Here's how the part is built. I have some questions about the finished solid (model axes, mm). A direction names the side the tool comes from. Give positions to 0.01 mm unless a question says otherwise; leave off trailing zeros. Loops run counter-clockwise (first coordinate to the right, second up) from the corner with the lowest first, then second, coordinate; pieces in that order, holes last. Notation, with made-up numbers: M 77.25,-4.75 L 86.25,-4.75 A17 cw 86.25,20.25 Z; hole C 34.25,-2.75 d2. An arc over 180 degrees is marked long. Answer as CSV lines item,"result". Start each with the question number.
Item 1: If I drill on line 1 along Y through (x, z) = (1, -1.75); line 2 along Y through (x, z) = (-0.75, 2); line 3 along Y through (x, z) = (4, -5), over which ranges is the centre line in solid material (lowest first)? Write a range as from..to.
Item 2: I want a section at D-D on y = 5.25. List the corners of the cut face in (x, z) for me.
Item 3: For faces 1 (the flat face through (-1.9, 7, 0)), 2 (the flat face through (-5.5, 1.6, -5.5)), which set-ups out of +Z, -Z, +X, -X, +Y, -Y let a thin tool reach every point of the face, with its end or its side?
Item 4: I want a section at A-A on z = 0. List the corners of the cut face in (x, y) for me.
Item 5: Will these pins go through, and if not, where does the flat tip stop? P1, Ø3, axis at x = -1, z = 0.5, coming from the -Y side; P2, Ø1.2, axis at x = -6.5, y = 0, coming from the -Z side; P3, Ø0.7, axis at x = 0, y = 5.5, coming from the +Z side.
Item 6: I want a section at B-B on x = 0. List the corners of the cut face in (y, z) for me, plus the area to 3 significant figures.
Item 7: I want a section at C-C on y = 0.5. List the corners of the cut face in (x, z) for me, plus the area to 3 significant figures.
Item 8: If we mould it in two halves opening along Y, with no side actions, what happens to faces 3 (the flat face through (3, 3.3, -3)), 4 (the flat face through (-1.6, 5, 0)), 5 (the flat face through (0, 0, 0)), 6 (the cylindrical face through (-2.038, 3.99, -2.658))? For each: released by +Y, released by -Y, zero draft, split by the parting line, or undercut.
from build123d import *

# Parameters (mm, degrees)
BOSS_EXTRUDE1_DEPTH = 3.3
BOSS_EXTRUDE2_START = 3.3
SKETCH3_R           = 3.35
BOSS_EXTRUDE2_DEPTH = 1.4
BOSS_EXTRUDE3_START = 4.7
SKETCH3_3_W         = 3.2
SKETCH3_3_H         = 3.2
BOSS_EXTRUDE3_DEPTH = 1.4
BOSS_EXTRUDE4_START = 6.1
SKETCH3_4_W         = 3.8
SKETCH3_4_H         = 3.8
BOSS_EXTRUDE4_DEPTH = 1.2
BOSS_EXTRUDE5_START = 2.5
BOSS_EXTRUDE5_DEPTH = 1
BOSS_EXTRUDE6_START = -2.5
BOSS_EXTRUDE6_DEPTH = 1


with BuildPart() as part:
    # Sketch1 → Boss-Extrude1 (new body)
    with BuildSketch(Plane(origin=(0, 0, 0), x_dir=(1, 0, 0), z_dir=(0, 1, 0))):
        Polygon((-5, 6), (-6, 5), (-6, -5), (-5, -6), (5, -6), (6, -5), (6, 5), (5, 6), align=None)
    extrude(amount=BOSS_EXTRUDE1_DEPTH)

    # Sketch3 → Boss-Extrude2 (add)
    with BuildSketch(Plane(origin=(0, 0, 0), x_dir=(1, 0, 0), z_dir=(0, 1, 0)).offset(BOSS_EXTRUDE2_START)):
        with Locations(Location((0, 0, 0), (0, 0, 270))):
            Circle(SKETCH3_R)
    extrude(amount=BOSS_EXTRUDE2_DEPTH)

    # Sketch3<3> → Boss-Extrude3 (add)
    with BuildSketch(Plane(origin=(0, 0, 0), x_dir=(1, 0, 0), z_dir=(0, 1, 0)).offset(BOSS_EXTRUDE3_START)):
        Rectangle(SKETCH3_3_W, SKETCH3_3_H)
    extrude(amount=BOSS_EXTRUDE3_DEPTH)

    # Sketch3<4> → Boss-Extrude4 (add)
    with BuildSketch(Plane(origin=(0, 0, 0), x_dir=(1, 0, 0), z_dir=(0, 1, 0)).offset(BOSS_EXTRUDE4_START)):
        Rectangle(SKETCH3_4_W, SKETCH3_4_H)
    extrude(amount=BOSS_EXTRUDE4_DEPTH)

    # Sketch4 → Boss-Extrude5 (add)
    with BuildSketch(Plane.XY.offset(BOSS_EXTRUDE5_START)):
        Polygon((6, 1.543469882), (7.05, -1.890925367), (6.35, -3.028306733), (6.35, -3.5), (6.25, -3.5), (6.25, -3), (6.941165312, -1.876973505), (6, 1.20143952), align=None)
        Polygon((-6.941165312, -1.876973505), (-6, 1.20143952), (-6, 1.543469882), (-7.05, -1.890925367), (-6.35, -3.028306733), (-6.35, -3.5), (-6.25, -3.5), (-6.25, -3), align=None)
    extrude(amount=BOSS_EXTRUDE5_DEPTH)

    # Sketch4<2> → Boss-Extrude6 (add)
    with BuildSketch(Plane.XY.offset(BOSS_EXTRUDE6_START)):
        Polygon((6, 1.543469882), (7.05, -1.890925367), (6.35, -3.028306733), (6.35, -3.5), (6.25, -3.5), (6.25, -3), (6.941165312, -1.876973505), (6, 1.20143952), align=None)
        Polygon((-6.941165312, -1.876973505), (-6, 1.20143952), (-6, 1.543469882), (-7.05, -1.890925367), (-6.35, -3.028306733), (-6.35, -3.5), (-6.25, -3.5), (-6.25, -3), align=None)
    extrude(amount=-BOSS_EXTRUDE6_DEPTH)


solid = part.part
Result:
1,line 1,"0..4.7, 6.1..7.3"
1,line 2,"0..4.7"
1,line 3,"0..3.3"
2,outline,"M -1.6,-1.6 L 1.6,-1.6 L 1.6,1.6 L -1.6,1.6 Z"
3,face 1,"+Z, -Z, -X, +Y"
3,face 2,"-Z, -X, +Y, -Y"
4,outline,"M -6,0 L 6,0 L 6,3.3 L 3.35,3.3 L 3.35,4.7 L 1.6,4.7 L 1.6,6.1 L 1.9,6.1 L 1.9,7.3 L -1.9,7.3 L -1.9,6.1 L -1.6,6.1 L -1.6,4.7 L -3.35,4.7 L -3.35,3.3 L -6,3.3 Z"
5,P1,"y = 0"
5,P2,"z = -5.1"
5,P3,"z = 1.6"
6,outline,"M 0,-6 L 3.3,-6 L 3.3,-3.35 L 4.7,-3.35 L 4.7,-1.6 L 6.1,-1.6 L 6.1,-1.9 L 7.3,-1.9 L 7.3,1.9 L 6.1,1.9 L 6.1,1.6 L 4.7,1.6 L 4.7,3.35 L 3.3,3.35 L 3.3,6 L 0,6 Z"
6,area,"58.0 mm^2"
7,outline,"M -6.32,-3.5 L -6.21,-3.5 L -6.21,-2.5 L -6.32,-2.5 Z; M -6.32,2.5 L -6.21,2.5 L -6.21,3.5 L -6.32,3.5 Z; M -6,-5 L -5,-6 L 5,-6 L 6,-5 L 6,5 L 5,6 L -5,6 L -6,5 Z; M 6.21,-3.5 L 6.32,-3.5 L 6.32,-2.5 L 6.21,-2.5 Z; M 6.21,2.5 L 6.32,2.5 L 6.32,3.5 L 6.21,3.5 Z"
7,area,"142 mm^2"
8,face 3,"released by +Y"
8,face 4,"undercut"
8,face 5,"released by -Y"
8,face 6,"zero draft"
